Input: part model. Units: mm. Frame: model coordinates. A direction names the side the tool comes from. Give positions to 0.01 mm unless a question says otherwise; leave off trailing zeros.
from build123d import *

# Parameters (mm, degrees)
F3_DEPTH = 6.986
F5_DEPTH = 3.175
F5_TAPER = 3
F7_D     = 4.064
F8_R     = 5.08


with BuildPart() as f1:
    # F0 (on Right) → F1 (revolve)
    with BuildSketch(Plane.YZ):
        with BuildLine():
            Line((0, 6.985), (0, 0))
            Line((0, 0), (25.4, 0))
            Line((25.4, 0), (25.4, 1.27))
            ThreePointArc((25.4, 1.27), (23.1775, 3.4925), (25.4, 5.715))
            Line((25.4, 5.715), (25.4, 6.985))
            Line((25.4, 6.985), (0, 6.985))
        make_face()
    revolve(axis=Axis((0, 0, 3.4925), (0, 0, -1)))

    # F2 (on face) → F3 (cut, through all)
    with BuildSketch(Plane(origin=(0, 0, 0), x_dir=(1, 0, 0), z_dir=(0, 0, -1))):
        with BuildLine():
            Line((0.2169925916, 12.6803131585), (1.5794517729, 22.1688059466))
            ThreePointArc((1.5794517729, 22.1688059466), (-10.3752942251, 19.6546151004), (-19.1953566714, 11.2021831469))
            Line((-19.1953566714, 11.2021831469), (-10.5922868167, 6.9743019418))
            Line((-10.5922868167, 6.9743019418), (0.2169925916, 12.6803131585))
        make_face()
        with BuildLine():
            Line((12.1267488565, 3.7120600417), (21.5718647936, 5.3483898817))
            ThreePointArc((21.5718647936, 5.3483898817), (15.4865075293, 15.9411012651), (4.722217854, 21.7175340115))
            Line((4.722217854, 21.7175340115), (3.3597586727, 12.2290412234))
            Line((3.3597586727, 12.2290412234), (12.1267488565, 3.7120600417))
        make_face()
        with BuildLine():
            ThreePointArc((11.7526938703, -18.8633192146), (19.4313438324, -10.787655068), (22.225, 0))
            ThreePointArc((22.225, 0), (22.1971945583, 1.1113859542), (22.1138478075, 2.2199910241))
            Line((22.1138478075, 2.2199910241), (12.6687318704, 0.5836611841))
            Line((12.6687318704, 0.5836611841), (7.2777503747, -10.3861338845))
            Line((7.2777503747, -10.3861338845), (11.7526938703, -18.8633192146))
        make_face()
        with BuildLine():
            ThreePointArc((-14.3083005224, -17.006562297), (-3.1589035458, -21.9993625678), (8.9448917131, -20.3455041039))
            Line((8.9448917131, -20.3455041039), (4.4699482176, -11.8683187738))
            Line((4.4699482176, -11.8683187738), (-7.6288517633, -10.131043794))
            Line((-7.6288517633, -10.131043794), (-14.3083005224, -17.006562297))
        make_face()
        with BuildLine():
            ThreePointArc((-20.5957099144, 8.3526856833), (-21.8987920037, -3.7938810973), (-16.5856007031, -14.7942040785))
            Line((-16.5856007031, -14.7942040785), (-9.906151944, -7.9186855756))
            Line((-9.906151944, -7.9186855756), (-11.9926400596, 4.1248044782))
            Line((-11.9926400596, 4.1248044782), (-20.5957099144, 8.3526856833))
        make_face()
    extrude(amount=-F3_DEPTH, mode=Mode.SUBTRACT)

    # F4 (on face) → F5 (join)
    with BuildSketch(Plane.XY.offset(6.985)):
        Polygon((9.7145011491, -5.157127827), (9.3234542833, 5.8344408667), (-0.3910468658, 10.9915686937), (-9.7145011491, 5.157127827), (-9.3234542833, -5.8344408667), (0.3910468658, -10.9915686937), align=None)
        Polygon((-6.7353874634, 3.5756086268), (-0.2711258269, 7.620820961), (6.4642616364, 4.0452123342), (6.7353874634, -3.5756086268), (0.2711258269, -7.620820961), (-6.4642616364, -4.0452123342), align=None, mode=Mode.SUBTRACT)
    extrude(amount=F5_DEPTH, taper=F5_TAPER)

    # F7 (through all)
    with Locations(Plane.XY.offset(6.985)):
        with Locations((0, 0)):
            Hole(F7_D / 2)

    # F8
    f8_edges = [f1.edges().sort_by_distance(p)[0] for p in [
        (-11.99264, -4.124804, 3.4925),
        (-9.906152, 7.918686, 3.4925),
        (4.469948, 11.868319, 3.4925),
        (0.216993, -12.680313, 3.4925),
        (7.27775, 10.386134, 3.4925),
        (12.668732, -0.583661, 3.4925),
        (3.359759, -12.229041, 3.4925),
        (12.126749, -3.71206, 3.4925),
        (-7.628852, 10.131044, 3.4925),
        (-10.592287, -6.974302, 3.4925),
    ]]
    fillet(f8_edges, radius=F8_R)


solid = f1.part
(1) Reachability of faces 1 (the flat face through (-1, 2, 6.985)), 2 (the cylindrical face through (4.085, 12.357, 3.541)) from +Z, -Z, +X, -X, +Y, -Y: full face, straight path, thin tool, end or side. Return the list, or none.
Values follow:
face 1: +Z
face 2: +Z, -Z
(2) Pin query (flat end, axial travel): pin 1 Ø6 at (y, z) = (-15.5, 8.5) entering from -X; pin 2 Ø2 at (y, z) = (-17, 4) entering from -X; pin 3 Ø6.5 at (x, y) = (2, -1) entering from +Z (3 decimals); pin 4 Ø1 at (x, y) = (-9, 5.5) entering from +Z. Return the tip coordinate at first contact, or that it passes through.
Values follow:
pin 1: stops at x = -21.87
pin 2: stops at x = -16.99
pin 3: stops at z = 6.985
pin 4: stops at z = 10.16
(3) Mould query, pull axis Y, two halves, no side actions, for faces 3 (the cylindrical face through (12.278, -4.316, 3.541)), 4 (the flat face through (10.1, 15.73, 3.44)), 5 (the flat face through (-7.4, 7.4, 6.985)). Classes: +Y half, -Y half, draft (parallel to the pull), parting line (faces both ways), or undercut.
Values follow:
face 3: undercut
face 4: undercut
face 5: draft
(4) Ray query, probe 1 along Y at (x, z) = (-16, 6.5); probe 2 along Y at (x, z) = (11, 5); probe 3 along Y at (x, z) = (-1, 3.5). Return the intervals inside material, ascending.
Values follow:
probe 1: y = -19.73 to -15.43, -9.63 to -6.09, 14.19 to 19.73
probe 2: y = -21.07 to -19.31, -4.93 to 2.81, 17.44 to 21.07
probe 3: y = -23.16 to -22.2, -12.23 to -1.77, 1.77 to 11.08, 22.2 to 23.16
(5) Cut plane A-A (z = 3). Count the separate pieces of the cut face and the enclosed holes in it, and give its area (3 significant figures).
Values follow:
separate pieces: 1
enclosed holes: 6
area: 733 mm2
